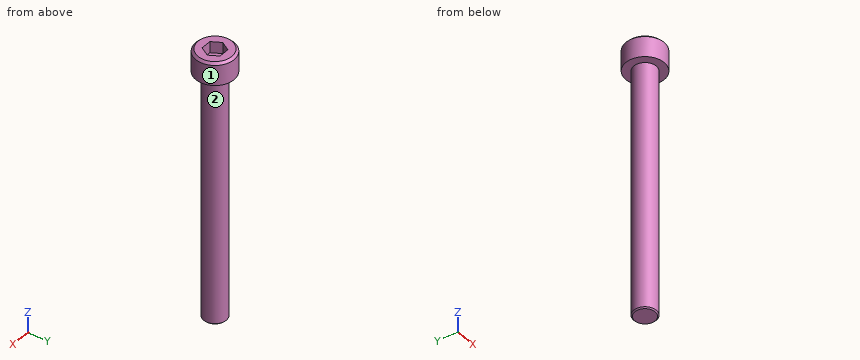
Autodesk Inventor part; units mm, degrees
ref_plane "YZ Plane" through (0, 0, 0) normal (1, 0, 0) x (0, 1, 0)
ref_plane "XZ Plane" through (0, 0, 0) normal (0, 1, 0) x (-1, 0, 0)
ref_plane "XY Plane" through (0, 0, 0) normal (0, 0, 1) x (1, 0, 0)
sketch "Sketch3" plane through (0, 0, 0) normal (0, 0, 1) x (1, 0, 0)
  circle A0 centre (0, 0) radius 2.5
  dimension "Diameter" = 5
extrude "Extrusion1" add sketch "Sketch3" against normal blind 55
sketch "Sketch4" plane through (0, 0, 0) normal (0, 0, 1) x (1, 0, 0)
  circle A0 centre (0, 0) radius 2.5
  circle A1 centre (0, 0) radius 4.25
  dimension "Head_Diameter" = 8.5
extrude "Extrusion2" add sketch "Sketch4" along normal blind 5 contours A0 | A1
sketch "Sketch5" plane through (0, 0, 5) normal (0, 0, 1) x (1, 0, 0)
  circle A0 centre (0, 0) radius 4.25
  line L0 (2.3094, 0) -> (1.1547, -2)
  line L1 (1.1547, -2) -> (-1.1547, -2)
  line L2 (-1.1547, -2) -> (-2.3094, 0)
  line L3 (-2.3094, 0) -> (-1.1547, 2)
  line L4 (-1.1547, 2) -> (1.1547, 2)
  line L5 (1.1547, 2) -> (2.3094, 0)
  line L6 (0, 0) -> (2.3094, 0) construction
  dimension "Hex_Width" = 4
extrude "Extrusion3" cut sketch "Sketch5" against normal blind 2.5 contours L0 L1 L2 L3 L4 L5
thread "Thread1"
chamfer "Chamfer1" distance 0.5 angle 45 1 edges at (-4.25, 0, 5)
chamfer "Chamfer2" distance 0.25 angle 45 1 edges at (-2.5, 0, -55)
equation "\"d14\" = 0.5 * Chamfer"
properties part number "fmpshma050080050" material "Steel, MS"
Verification items for the finished model (mm, model axes). Face numbers are marked on the shaded views. A direction names the side the tool comes from. Give positions to 0.01 mm unless a question says otherwise; leave off trailing zeros. Loops run counter-clockwise (first coordinate to the right, second up) from the corner with the lowest first, then second, coordinate; pieces in that order, holes last.
1. Cross-section at B-B on z = -10.5. Record the cut outline in (x, y).
Derived:
outline: circle Ø5 at (0, 0)
2. Material ranges on probe 1 along Z at (x, y) = (-1.25, 2.25); probe 2 along X at (y, z) = (1.5, -47); probe 3 along Y at (x, z) = (0, -20.5), recorded low to high.
Derived:
probe 1: z = 0 to 5
probe 2: x = -2 to 2
probe 3: y = -2.5 to 2.5
3. Tool access check on the marked faces 1 and 2. Record the directions out of +Z, -Z, +X, -X, +Y, -Y that give a thin tool (end or side, any length) a straight path to the whole face; none if there is none.
Derived:
face 1: +Z, -Z
face 2: -Z
4. Cross-section at A-A on x = 0. Record the cut outline in (y, z), and give its area (3 significant figures).
Derived:
outline: (-4.25, 0) - (-2.5, 0) - (-2.5, -54.75) - (-2.25, -55) - (2.25, -55) - (2.5, -54.75) - (2.5, 0) - (4.25, 0) - (4.25, 4.5) - (3.75, 5) - (2, 5) - (2, 2.5) - (-2, 2.5) - (-2, 5) - (-3.75, 5) - (-4.25, 4.5) - close
area: 307 mm2
5. Go/stop test with flat-tipped pins: P1, Ø1.2, axis at x = 0.5, y = -0.5, coming from the +Z side; P2, Ø3, axis at y = -1, z = -3.5, coming from the -X side; P3, Ø2, axis at y = -0.5, z = -41, coming from the +X side; P4, Ø1.2, axis at x = -0.5, z = 3.5, coming from the -Y side. Record where each tip stops, or that it passes through.
Derived:
P1: stops at z = 2.5
P2: stops at x = -2.5
P3: stops at x = 2.5
P4: stops at y = -4.25
